from build123d import *

# Parameters (mm, degrees)
SKETCH1_RX          = 16
SKETCH1_RY          = 12
BOSS_EXTRUDE1_DEPTH = 0.9
BOSS_EXTRUDE2_DEPTH = 6
SKETCH4_R           = 3
CUT_EXTRUDE1_DEPTH  = 10
SKETCH5_RX          = 15
SKETCH5_RY          = 11
BOSS_EXTRUDE3_DEPTH = 1.7
SKETCH6_RX          = 16
SKETCH6_RY          = 12
BOSS_EXTRUDE4_DEPTH = 0.9


with BuildPart() as part:
    # Sketch1 → Boss-Extrude1 (new body)
    with BuildSketch(Plane(origin=(0, 0, 0), x_dir=(1, 0, 0), z_dir=(0, 1, 0))):
        with Locations(Location((0, 0), (0, 0, 90))):
            Ellipse(SKETCH1_RX, SKETCH1_RY)
    extrude(amount=BOSS_EXTRUDE1_DEPTH)

    # Sketch3 → Boss-Extrude2 (add)
    with BuildSketch(Plane(origin=(0, 0, 0), x_dir=(-1, 0, 0), z_dir=(0, -1, 0))):
        with BuildLine():
            ThreePointArc((12.379824796, -4.986278203), (17.749999782, -0.001477913), (12.382772576, 4.986496167))
            ThreePointArc((12.382772576, 4.986496167), (5.304706978, 5.301894868), (4.986278203, 12.379824796))
            ThreePointArc((4.986278203, 12.379824796), (0.001477913, 17.749999782), (-4.986496167, 12.382772576))
            ThreePointArc((-4.986496167, 12.382772576), (-5.301894868, 5.304706978), (-12.379824796, 4.986278203))
            ThreePointArc((-12.379824796, 4.986278203), (-17.749999782, 0.001477913), (-12.382772576, -4.986496167))
            ThreePointArc((-12.382772576, -4.986496167), (-5.304706978, -5.301894868), (-4.986278203, -12.379824796))
            ThreePointArc((-4.986278203, -12.379824796), (-0.001477913, -17.749999782), (4.986496167, -12.382772576))
            ThreePointArc((4.986496167, -12.382772576), (5.301894868, -5.304706978), (12.379824796, -4.986278203))
        make_face()
    extrude(amount=BOSS_EXTRUDE2_DEPTH)

    # Sketch4 → Cut-Extrude1 (cut)
    with BuildSketch(Plane(origin=(0, 0.9, 0), x_dir=(1, 0, 0), z_dir=(0, 1, 0))):
        Circle(SKETCH4_R)
    extrude(amount=-CUT_EXTRUDE1_DEPTH, mode=Mode.SUBTRACT)

    # Sketch5 → Boss-Extrude3 (add)
    with BuildSketch(Plane(origin=(0, 0.9, 0), x_dir=(1, 0, 0), z_dir=(0, 1, 0))):
        with Locations(Location((0, 0), (0, 0, 90))):
            Ellipse(SKETCH5_RX, SKETCH5_RY)
    extrude(amount=BOSS_EXTRUDE3_DEPTH)

    # Sketch6 → Boss-Extrude4 (add)
    with BuildSketch(Plane(origin=(0, 2.6, 0), x_dir=(1, 0, 0), z_dir=(0, 1, 0))):
        with Locations(Location((0, 0), (0, 0, 90))):
            Ellipse(SKETCH6_RX, SKETCH6_RY)
    extrude(amount=BOSS_EXTRUDE4_DEPTH)


solid = part.part
Could you check a few things on this model? Use its own coordinates, in mm. A direction names the side the tool comes from. Give positions to 0.01 mm unless a question says otherwise; leave off trailing zeros. Order: outer loops, then holes, each group sorted by start corner. A loop starts at its lowest first (then second) coordinate and runs counter-clockwise, first axis right, second up. Notation, with made-up numbers: (78, -12.5) - (110, -12.5) arc R18 cw to (110, 1.5) - close; hole circle Ø9 at (-12.75, -9). An arc over 180 degrees is marked (long way). One line per item, written item: value. Start each with the question number.
1. If I drill on probe 1 along Z at (x, y) = (0, -2.25); probe 2 along Y at (x, z) = (-6, 13.5), over which ranges is the centre line in solid material (lowest first)?
2. For faces 4 (the face through (0, -6, 4)), 5 (the face through (0, 0, -17)), 6 (the face through (-5.23, -2.96, 5.38)), 7 (the face through (-11, 2.6, -3)), which set-ups out of +Z, -Z, +X, -X, +Y, -Y let a thin tool reach every point of the face, with its end or its side?
3. For P1, Ø3, axis at x = -15.5, z = 1, coming from the +Y side; P2, Ø2.5, axis at x = -6.5, z = 10.5, coming from the -Y side; P3, Ø4, axis at y = -0.5, z = -8.5, coming from the -X side, each with a flat end and sliding along its axis, tell me the tip position at first contact or that it passes through.
4. Imagine slicing it at B-B on x = 14. List the corners of the cut face in (y, z) for me.
5. Thinking about a two-plate mould opening in X: for faces 1 (the face through (-8, 0, -8)), 2 (the face through (0, 3.5, 0)), 3 (the face through (0.12, -2.96, 17.75)), which applies, +X half, -X half, draft (parallel to the pull), parting line (faces both ways), or undercut?
Values:
1. probe 1: -17.75 to -3, 3 to 17.75
1. probe 2: 0 to 0.9, 2.6 to 3.5
2. face 4: +Z, -Z, +X, -X, -Y
2. face 5: -Z, +Y
2. face 6: -Y
2. face 7: none
3. P1: y = 0
3. P2: y = 0
3. P3: x = -10.94
4. outline: (-6, -4.84) - (0, -4.84) - (0, 4.84) - (-6, 4.84) - close
5. face 1: undercut
5. face 2: draft
5. face 3: parting line
